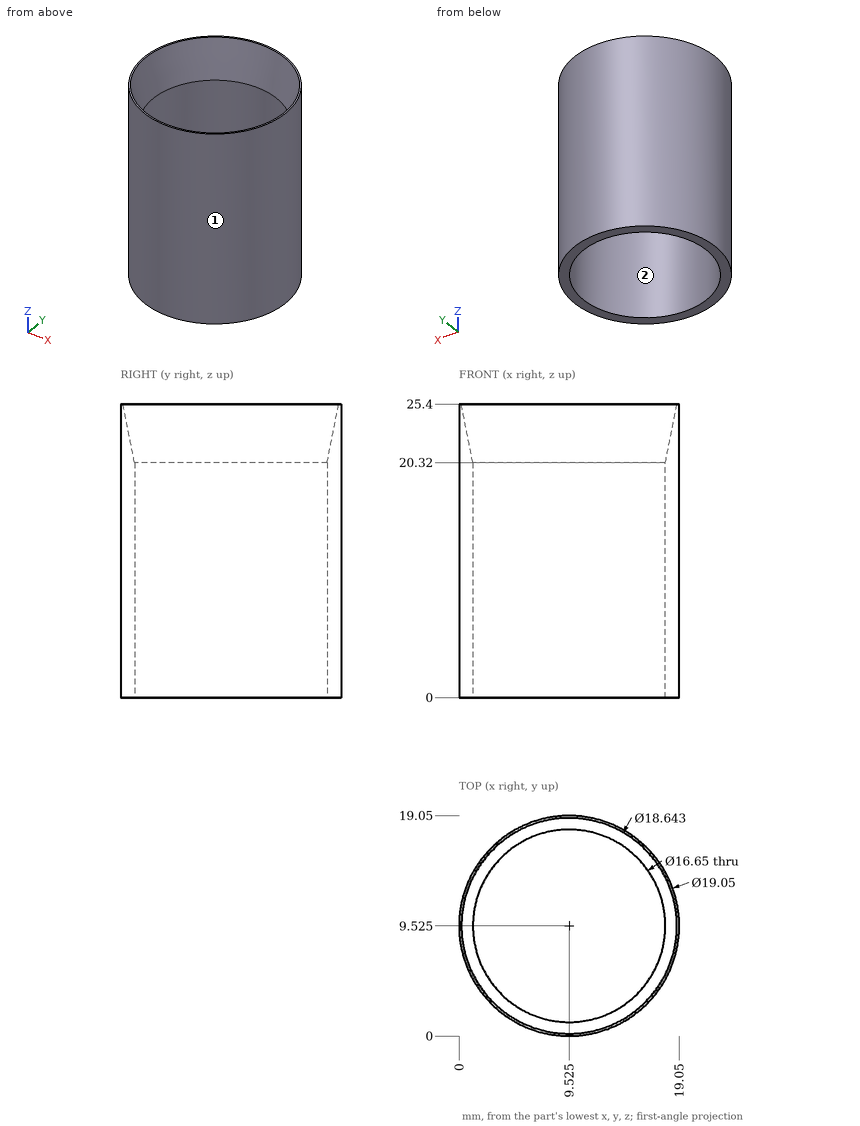
Verification items for this drawing (mm, ordinates from the low corner). Coordinates: 2 decimals unless noted, no trailing zeros.
Item 1: Release check for a two-part mould opening along Y. For the marked faces 1 and 2 record: released by +Y, released by -Y, zero draft, split by the parting line, or undercut.
Item 2: Go/stop test with flat-tipped pins: pin 1 Ø4 at (x, z) = (12.5, 16) entering from +Y; pin 2 Ø1 at (y, z) = (12, 9.5) entering from +X. Record where each tip stops, or that it passes through.
Item 3: Thickness scan on line 1 (Y direction, x = 9.25, z = 12) (1 decimal); line 2 (Y direction, x = 3.75, z = 11); line 3 (X direction, y = 5, z = 1.75). Record the ranges inside material, lowest first.
Check result:
1. face 1: split by the parting line
1. face 2: undercut
2. pin 1: stops at y = 19
2. pin 2: stops at x = 18.84
3. line 1: y = 0 to 1.2, 17.8 to 19
3. line 2: y = 1.95 to 3.53, 15.52 to 17.1
3. line 3: x = 1.14 to 2.54, 16.51 to 17.91
